CAD build for the part. Positions are in the model's coordinates, mm. A direction names the side the tool comes from. Round coordinates to 2 decimals unless told otherwise and drop trailing zeros. Loops run counter-clockwise (first coordinate to the right, second up) from the corner with the lowest first, then second, coordinate; pieces in that order, holes last.
from build123d import *

# Parameters (mm, degrees)
F0_W     = 75
F0_H     = 4
F5_DEPTH = 25


with BuildPart() as f1:
    # F0 (on Top) → F1 (revolve)
    with BuildSketch(Plane.XY):
        with Locations((12.5, 12)):
            Rectangle(F0_W, F0_H)
    revolve(axis=Axis((-0.954778, 0, 0), (1, 0, 0)))

    # F2 (on Front) → F3 (revolve)
    with BuildSketch(Plane.XZ):
        Polygon((-6.970563, 12.828427), (-4.142136, 10), (21.389404, 35.53154), (28.460472, 28.460472), (37.413038, 37.413038), (30.45914, 44.601276), (27.67767, 41.819805), (22.316322, 47.181152), (13.123934, 37.988764), (12.828427, 32.627416), align=None)
    revolve(axis=Axis((18.706519, 0, 18.706519), (0.707107, 0, 0.707107)))

    # F4 (on face) → F5 (cut)
    with BuildSketch(Plane(origin=(34.748737, 0, 34.748737), x_dir=(0.707107, 0, -0.707107), z_dir=(0.707107, 0, 0.707107))):
        Polygon((7, -4.041452), (7, 4.041452), (0, 8.082904), (-7, 4.041452), (-7, -4.041452), (0, -8.082904), align=None)
    extrude(amount=F5_DEPTH, mode=Mode.SUBTRACT)


solid = f1.part
Item 1: 3-axis set-ups, long thin cutter, end or side, ignore diameter. For faces 4 (the flat face through (41.1, -0.1, 31.2)), 5 (the flat face through (33.67, 6.09, 38.55)), 6 (the flat face through (-25, 3, 10)), 7 (the cylindrical face through (15.6, -0.2, 1.46)): which of +Z, -Z, +X, -X, +Y, -Y reach the whole face in a straight line?
Verdict:
face 4: +Z
face 5: none
face 6: +Z, -Z, -X, +Y, -Y
face 7: -X
Item 2: Flat gauge pins, fed straight in: P1, Ø8, axis at y = -9, z = 15, coming from the +X side; P2, Ø2, axis at x = 1.5, z = 23.5, coming from the -Y side; P3, Ø5, axis at x = 34, y = 3.5, coming from the -Z side; P4, Ø18, axis at y = 0, z = 0, coming from the -X side. Where does each tip first touch, or does it go through?
Verdict:
P1: stops at x = 50
P2: passes through
P3: stops at z = -13.96
P4: stops at x = 6.01
Item 3: Wall check: L1, parallel to Z at x = 31, y = 6; L2, parallel to Z at x = 5, y = 0; L3, parallel to Z at x = -13, y = -8. Give the ranges that are in metal, low to high.
Verdict:
L1: z = -12.65 to -8, 8 to 12.65, 13.11 to 19.69, 25.92 to 42.31
L2: z = -14 to -10, 10 to 14, 19.14 to 24.8
L3: z = -11.49 to -6, 6 to 11.49
Item 4: Mould opens along Z. For faces 1 (the flat face through (50, 3, 10)), 2 (the flat face through (10.48, -0.14, -4.62)), 3 (the conical face through (42.575, -0.316, 32.42)) say: released by +Z, released by -Z, zero draft, split by the parting line, or undercut.
Verdict:
face 1: zero draft
face 2: undercut
face 3: released by +Z
Item 5: Cut at B-B (x = -20). List the corners of the cut face in (y, z).
Verdict:
outline: circle Ø28 at (0, 0); hole circle Ø20 at (0, 0)
Item 6: Cut at A-A (y = 0). State how many separate pieces and enclosed holes the cut face has, plus the area to 3 significant figures.
Verdict:
separate pieces: 2
enclosed holes: 1
area: 1,230 mm2
